```python
from build123d import *

# Parameters (mm, degrees)
SKETCH1_W           = 750
SKETCH1_H           = 50.8
SKETCH1_R           = 6.35
BOSS_EXTRUDE1_DEPTH = 50.8
SKETCH2_R           = 6.35
BOSS_EXTRUDE2_DEPTH = 12.7


with BuildPart() as part:
    # Sketch1 → Boss-Extrude1 (new body)
    with BuildSketch(Plane.XY):
        with Locations((335.619050288, -16.370527994)):
            Rectangle(SKETCH1_W, SKETCH1_H)
        with Locations((10.619050288, -16.370527994)):
            Circle(SKETCH1_R, mode=Mode.SUBTRACT)
    extrude(amount=BOSS_EXTRUDE1_DEPTH)

    # Sketch2 → Boss-Extrude2 (add)
    with BuildSketch(Plane.XY.offset(50.8)):
        with Locations((310.619050288, -16.370527994)):
            Circle(SKETCH2_R)
    extrude(amount=BOSS_EXTRUDE2_DEPTH)


solid = part.part
```
Input: part model. Units: mm. Frame: model coordinates. Round coordinates to 2 decimals unless told otherwise and drop trailing zeros. Loops run counter-clockwise (first coordinate to the right, second up) from the corner with the lowest first, then second, coordinate; pieces in that order, holes last.
1) Pin query (flat end, axial travel): pin 1 (15 mm diameter, centred on x = 223, y = -23.5, fed in from +Z); pin 2 (11.5 mm diameter, centred on x = 10.62, y = -16.37, fed in from -Z). Return the tip coordinate at first contact, or that it passes through.
Ans:
pin 1: stops at z = 50.8
pin 2: passes through
2) Section query A-A on y = -32.5. Return the cut outline in (x, z), plus the area to 3 significant figures.
Ans:
outline: (-39.38, 0) - (710.62, 0) - (710.62, 50.8) - (-39.38, 50.8) - close
area: 38,100 mm2
3) Pull-direction query (X, two-part tool) for faces 1 (the flat face through (330, -16, 0)), 2 (the cylindrical face through (5.58, -20.234, 25.044)), 3 (the cylindrical face through (304.275, -16.091, 57.061)); classes: released by +X, released by -X, zero draft, split by the parting line, or undercut.
Ans:
face 1: zero draft
face 2: undercut
face 3: split by the parting line
4) Section query B-B on x = 240. Return the cut outline in (y, z).
Ans:
outline: (-41.77, 0) - (9.03, 0) - (9.03, 50.8) - (-41.77, 50.8) - close
5) Material intervals for line 1 (Z direction, x = 600, y = -32); line 2 (X direction, y = -10.5, z = 38.5); line 3 (X direction, y = -14, z = 17), sorted ascending.
Ans:
line 1: z = 0 to 50.8
line 2: x = -39.38 to 8.2, 13.04 to 710.62
line 3: x = -39.38 to 4.73, 16.51 to 710.62
